```python
from build123d import *

# Parameters (mm, degrees)
F0_W     = 440
F0_H     = 690
F0_W_2   = 340
F0_H_2   = 590
F1_DEPTH = 6
F2_W     = 100
F2_H     = 40
F2_W_2   = 340
F2_H_2   = 590
F3_DEPTH = 3


with BuildPart() as f1:
    # F0 (on Top) → F1 (new body)
    with BuildSketch(Plane.XY):
        with Locations((175, 300)):
            Rectangle(F0_W, F0_H)
        with Locations((175, 300)):
            Rectangle(F0_W_2, F0_H_2, mode=Mode.SUBTRACT)
    extrude(amount=F1_DEPTH)

    # F2 (on face) → F3 (cut)
    with BuildSketch(Plane(origin=(0, 0, 0), x_dir=(1, 0, 0), z_dir=(0, 0, -1))):
        with Locations((175, 20)):
            Rectangle(F2_W, F2_H)
        Polygon((0, -600), (350, -600), (350, 0), (225, 0), (125, 0), (0, 0), align=None)
        with Locations((175, -300)):
            Rectangle(F2_W_2, F2_H_2, mode=Mode.SUBTRACT)
    extrude(amount=-F3_DEPTH, mode=Mode.SUBTRACT)


solid = f1.part
```
Can you work these out from the model? Positions are in its coordinate system, mm. Coordinates: 2 decimals unless noted, no trailing zeros. Loops run counter-clockwise (first coordinate to the right, second up) from the corner with the lowest first, then second, coordinate; pieces in that order, holes last. Notation, with made-up numbers: M 28,44.25 L 76,44.25 A26 ccw 76,75.25 Z; hole C -17.5,-30.75 d8. An arc over 180 degrees is marked long. Put each result on its own line as item: value. Start each with the question number.
(1) Imagine slicing it at C-C on y = 556.5. List the corners of the cut face in (x, z) for me, and give its area (3 significant figures).
(2) I need wall thicknesses on probe 1 along X at (y, z) = (525.5, 2.1); probe 2 along Y at (x, z) = (272, 1.9); probe 3 along X at (y, z) = (35, 3.65). Which ranges of each line are inside material? Lowest first, please.
(3) We'd pull the mould along X, two halves only. Please class faces 1 (the face through (174, -6, 3)), 2 (the face through (-24, 305, 0)): +X half, -X half, draft (parallel to the pull), parting line (faces both ways), or undercut.
(4) Imagine slicing it at A-A on x = 61. List the corners of the cut face in (y, z) for me, and give its area (3 significant figures).
(5) Imagine slicing it at B-B on z = 4.2. List the corners of the cut face in (x, y) for me, and give its area (3 significant figures).
Worked answers:
1. outline: M -45,0 L 0,0 L 0,3 L 5,3 L 5,6 L -45,6 Z; M 345,3 L 350,3 L 350,0 L 395,0 L 395,6 L 345,6 Z
1. area: 570 mm2
2. probe 1: x = -45 to 0, 350 to 395
2. probe 2: y = -45 to 0, 600 to 645
2. probe 3: x = -45 to 5, 345 to 395
3. face 1: undercut
3. face 2: draft
4. outline: M -45,0 L 0,0 L 0,3 L 5,3 L 5,6 L -45,6 Z; M 595,3 L 600,3 L 600,0 L 645,0 L 645,6 L 595,6 Z
4. area: 570 mm2
5. outline: M -45,-45 L 395,-45 L 395,645 L -45,645 Z; hole M 5,5 L 345,5 L 345,595 L 5,595 Z
5. area: 103,000 mm2
